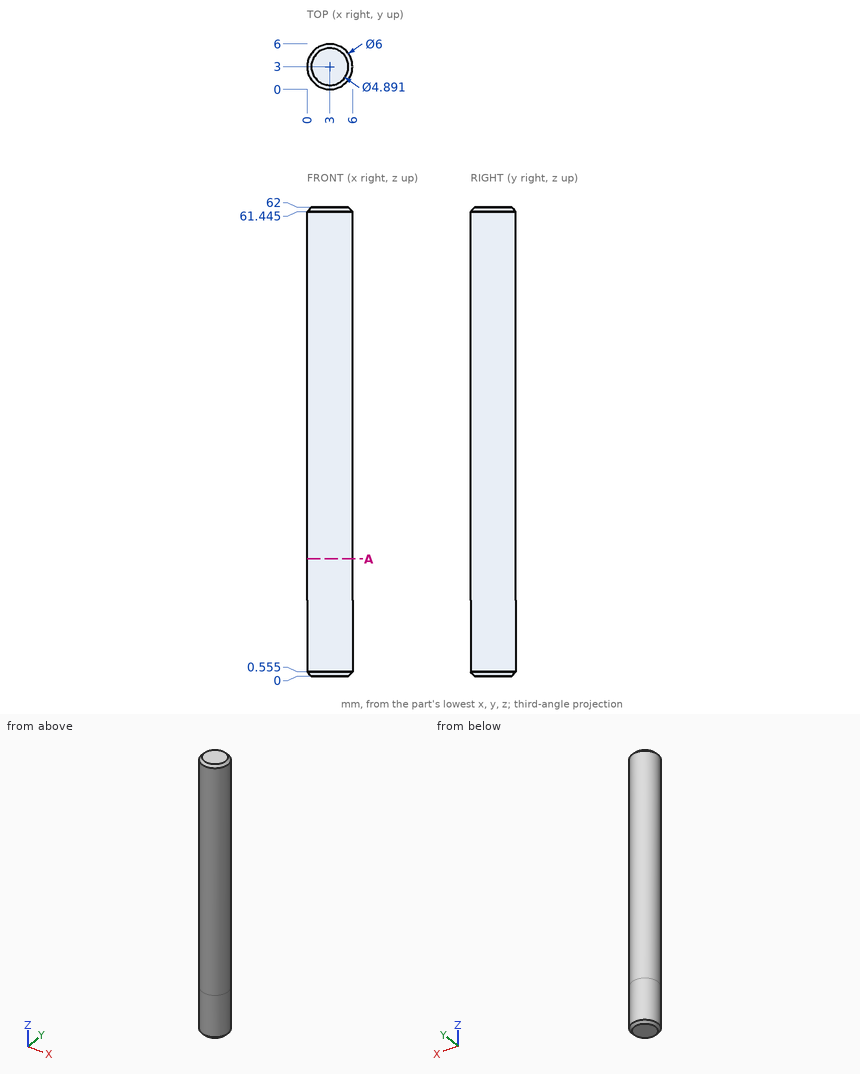
The drawing under review shows one solid part. Ordinate dimensions are in mm from its lowest x, y, z. Round coordinates to 2 decimals unless told otherwise and drop trailing zeros. Loops run counter-clockwise (first coordinate to the right, second up) from the corner with the lowest first, then second, coordinate; pieces in that order, holes last. Notation, with made-up numbers: M 37.5,23.25 L 43.5,23.25 A6 cw 43.5,27.25 Z; hole C 89,21 d7. An arc over 180 degrees is marked long. Answer as CSV lines item,"result". Start each with the question number.
Item 1: Wall thickness on line 1 (Y direction, x = 2.9, z = 38); line 2 (X direction, y = 5.25, z = 29.5) (1 decimal); line 3 (X direction, y = 2.5, z = 54): over which ranges is each line inside the solid? List them lowest first. Write a range as [from, to].
Item 2: Insertion check: P1, Ø2, axis at x = 2, z = 40.5, coming from the -Y side. The pin has a flat end and moves straight along its axis. Give the tip position at first contact, or say it passes through.
Item 3: Consider section A-A (z = 15.5). Write out the cut boundary in (x, y).
Answer:
1,line 1,"y = [0, 6]"
1,line 2,"x = [1, 5]"
1,line 3,"x = [0.04, 5.96]"
2,P1,"stops at y = 0"
3,outline,"C 3,3 d6"
